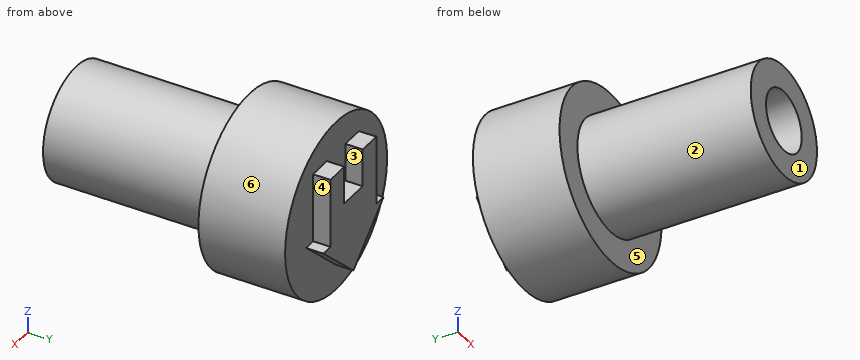
```python
from build123d import *

# Parameters (mm, degrees)
SKETCH1_R           = 3.25
BOSS_EXTRUDE1_DEPTH = 10
SKETCH2_R           = 1.75
CUT_EXTRUDE1_DEPTH  = 2.5
SKETCH6_R           = 5
BOSS_EXTRUDE2_DEPTH = 5
BOSS_EXTRUDE3_DEPTH = 1


with BuildPart() as part:
    # Sketch1 → Boss-Extrude1 (new body)
    with BuildSketch(Plane(origin=(0, 0, 0), x_dir=(1, 0, 0), z_dir=(0, 1, 0))):
        Circle(SKETCH1_R)
    extrude(amount=BOSS_EXTRUDE1_DEPTH)

    # Sketch2 → Cut-Extrude1 (cut)
    with BuildSketch(Plane.XZ):
        Circle(SKETCH2_R)
    extrude(amount=-CUT_EXTRUDE1_DEPTH, mode=Mode.SUBTRACT)

    # Sketch6 → Boss-Extrude2 (add)
    with BuildSketch(Plane(origin=(0, 10, 0), x_dir=(1, 0, 0), z_dir=(0, 1, 0))):
        Circle(SKETCH6_R)
    extrude(amount=BOSS_EXTRUDE2_DEPTH)

    # Sketch12 → Boss-Extrude3 (add)
    with BuildSketch(Plane(origin=(0, 15, 0), x_dir=(1, 0, 0), z_dir=(0, 1, 0))):
        Polygon((0, 3.542487974), (-2.95, 0.842487974), (-2.25, 0.842487974), (-2.25, -3.157512026), (-0.9, -3.172366953), (-0.9, -0.972366953), (0.9, -0.972366953), (0.9, -3.172366953), (2.25, -3.157512026), (2.25, 0.842487974), (2.95, 0.842487974), align=None)
    extrude(amount=BOSS_EXTRUDE3_DEPTH)


solid = part.part
```
Source: CAD feature listing. Evaluate the final solid. Frame: model axes, mm. Face numbers are marked on the shaded views. A direction names the side the tool comes from. Round coordinates to 2 decimals unless told otherwise and drop trailing zeros. Loops run counter-clockwise (first coordinate to the right, second up) from the corner with the lowest first, then second, coordinate; pieces in that order, holes last. Notation, with made-up numbers: M -18,31.25 L 32,31.25 A10 ccw 32,42.25 Z; hole C -8,-6 d9. An arc over 180 degrees is marked long. Use a Markdown table: item, result. Add a question column.
1. Section query D-D on z = 2.5. Return the cut outline in (x, y), then the cut area to 3 significant figures.
2. Reachability of the marked faces 4, 5 and 6 from +Z, -Z, +X, -X, +Y, -Y: full face, straight path, thin tool, end or side. Return the list, or none.
3. Mould query, pull axis X, two halves, no side actions, for the marked faces 1, 2 and 3. Classes: pulls with the +X half, pulls with the -X half, needs draft (parallel to the pull), parting line crosses it, or undercut.
4. Section query C-C on x = -3.5. Return the cut outline in (y, z), then the cut area to 3 significant figures.
5. Line query: line 1 (Z direction, x = 0, y = 1.7); line 2 (Y direction, x = -1.5, z = -3.5); line 3 (Z direction, x = -2.25, y = 11.25). Output: solid intervals per line, ascending.
6. Contact query for flat-ended pins moving along their axis: P1, Ø0.5, axis at y = 15.5, z = 1, coming from the +X side; P2, Ø3, axis at x = 0.5, z = 0, coming from the -Y side; P3, Ø6, axis at x = -2.5, y = 6, coming from the -Z side; P4, Ø0.8, axis at y = 15.5, z = 0.5, coming from the -X side. Output: stop coordinate, or through.
7. Section query A-A on z = 0. Return the cut outline in (x, y), then the cut area to 3 significant figures.
8. Section query B-B on y = 2.75. Return the cut outline in (x, z), then the cut area to 3 significant figures.
Reported:
| question | item | result |
|---|---|---|
| 1 | outline | M -4.33,10 L -2.08,10 L -2.08,0 L 2.08,0 L 2.08,10 L 4.33,10 L 4.33,15 L 2.25,15 L 2.25,16 L 0.9,16 L 0.9,15 L -0.9,15 L -0.9,16 L -2.25,16 L -2.25,15 L -4.33,15 Z |
| 1 | area | 87.5 mm² |
| 2 | face 4 | +Z, +X, +Y |
| 2 | face 5 | -Y |
| 2 | face 6 | +Y, -Y |
| 3 | face 1 | needs draft |
| 3 | face 2 | parting line crosses it |
| 3 | face 3 | undercut |
| 4 | outline | M 10,-3.57 L 15,-3.57 L 15,3.57 L 10,3.57 Z |
| 4 | area | 35.7 mm² |
| 5 | line 1 | z = -3.25 to -1.75, 1.75 to 3.25 |
| 5 | line 2 | y = 10 to 15 |
| 5 | line 3 | z = -4.47 to 4.47 |
| 6 | P1 | stops at x = 2.25 |
| 6 | P2 | stops at y = 0 |
| 6 | P3 | stops at z = -3.25 |
| 6 | P4 | stops at x = -2.25 |
| 7 | outline | M -5,10 L -3.25,10 L -3.25,0 L -1.75,0 L -1.75,2.5 L 1.75,2.5 L 1.75,0 L 3.25,0 L 3.25,10 L 5,10 L 5,15 L 2.25,15 L 2.25,16 L -2.25,16 L -2.25,15 L -5,15 Z |
| 7 | area | 111 mm² |
| 8 | outline | C 0,0 d6.5 |
| 8 | area | 33.2 mm² |
